Job drawing, mm, ordinate dimensions from the low corner. One solid piece. Give positions to 0.01 mm unless a question says otherwise; leave off trailing zeros. Order: outer loops, then holes, each group sorted by start corner. A loop starts at its lowest first (then second) coordinate and runs counter-clockwise, first axis right, second up.
1. Mould opens along Z. For the marked faces 1, 2 and 3 say: +Z half, -Z half, draft (parallel to the pull), parting line (faces both ways), or undercut.
2. Slice it at B-B on y = 7.5. List the corners of the cut face in (x, z), and give its area (3 significant figures).
3. Slice it at C-C on z = 55. List the corners of the cut face in (x, y), and give its area (4 significant figures).
4. Slice it at A-A on z = 17.5. List the corners of the cut face in (x, y).
5. Drop flat-ended pins along their axis: pin 1 Ø3 at (x, z) = (56.5, 114) entering from +Y; pin 2 Ø11 at (x, z) = (52.5, 11.5) entering from +Y; pin 3 Ø11 at (y, z) = (29.5, 150) entering from +X; pin 4 Ø5 at (x, z) = (66, 54) entering from -Y. Give the stop position or say it passes through.
6. Slice it at D-D on y = 29.5. Give the number of separate pieces and of enclosed holes in the cut face, and give its area (3 significant figures).
7. Probe line 1 (X direction, y = 31.5, z = 85); line 2 (Y direction, x = 86, z = 137.5); line 3 (X direction, y = 25.5, z = 89). List the from-to ranges inside material, lowest first.
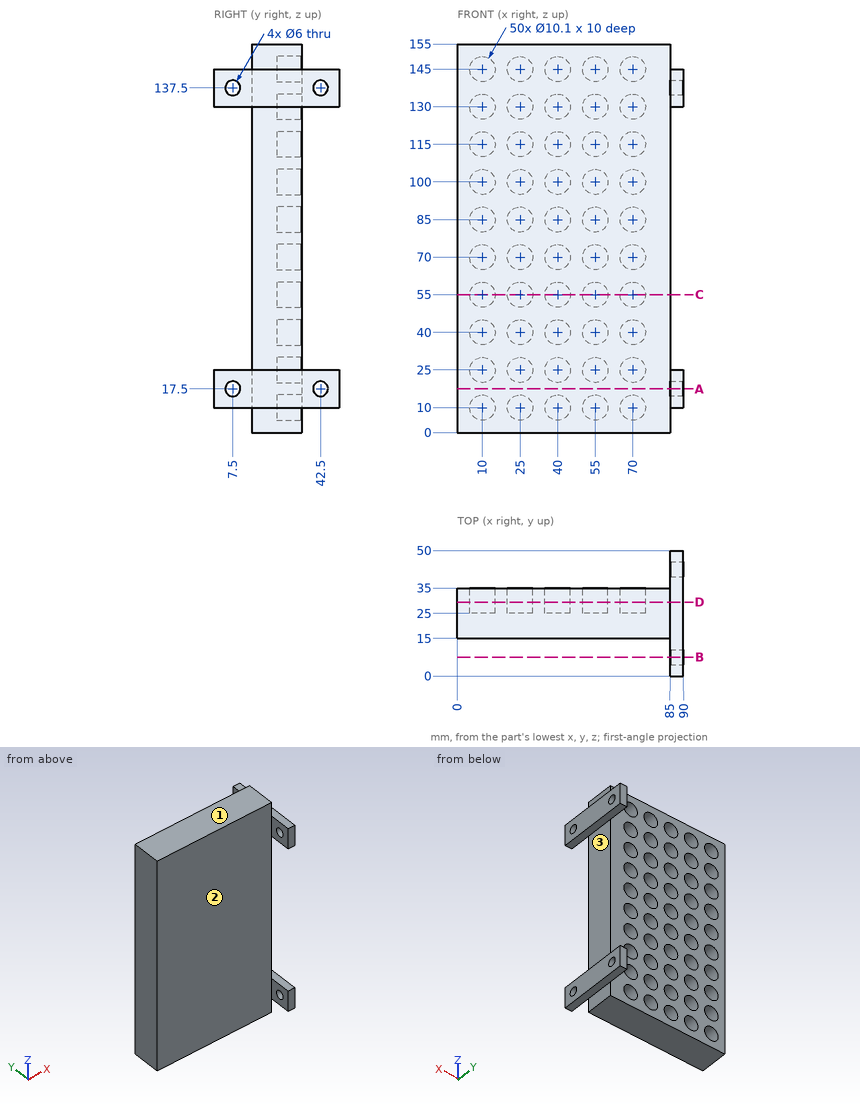
Data:
1. face 1: +Z half
1. face 2: draft
1. face 3: undercut
2. outline: (85, 10) - (90, 10) - (90, 14.5) - (85, 14.5) - close; (85, 20.5) - (90, 20.5) - (90, 25) - (85, 25) - close; (85, 130) - (90, 130) - (90, 134.5) - (85, 134.5) - close; (85, 140.5) - (90, 140.5) - (90, 145) - (85, 145) - close
2. area: 90.0 mm2
3. outline: (0, 15) - (85, 15) - (85, 35) - (75.05, 35) - (75.05, 25) - (64.95, 25) - (64.95, 35) - (60.05, 35) - (60.05, 25) - (49.95, 25) - (49.95, 35) - (45.05, 35) - (45.05, 25) - (34.95, 25) - (34.95, 35) - (30.05, 35) - (30.05, 25) - (19.95, 25) - (19.95, 35) - (15.05, 35) - (15.05, 25) - (4.95, 25) - (4.95, 35) - (0, 35) - close
3. area: 1,195 mm2
4. outline: (0, 15) - (85, 15) - (85, 10.5) - (90, 10.5) - (90, 39.5) - (85, 39.5) - (85, 35) - (0, 35) - close; (85, 0) - (90, 0) - (90, 4.5) - (85, 4.5) - close; (85, 45.5) - (90, 45.5) - (90, 50) - (85, 50) - close
5. pin 1: stops at y = 25
5. pin 2: stops at y = 35
5. pin 3: stops at x = 90
5. pin 4: stops at y = 15
6. separate pieces: 1
6. enclosed holes: 50
6. area: 9,320 mm2
7. line 1: x = 0 to 4.95, 15.05 to 19.95, 30.05 to 34.95, 45.05 to 49.95, 60.05 to 64.95, 75.05 to 85
7. line 2: y = 0 to 4.5, 10.5 to 39.5, 45.5 to 50
7. line 3: x = 0 to 6.92, 13.08 to 21.92, 28.08 to 36.92, 43.08 to 51.92, 58.08 to 66.92, 73.08 to 85
